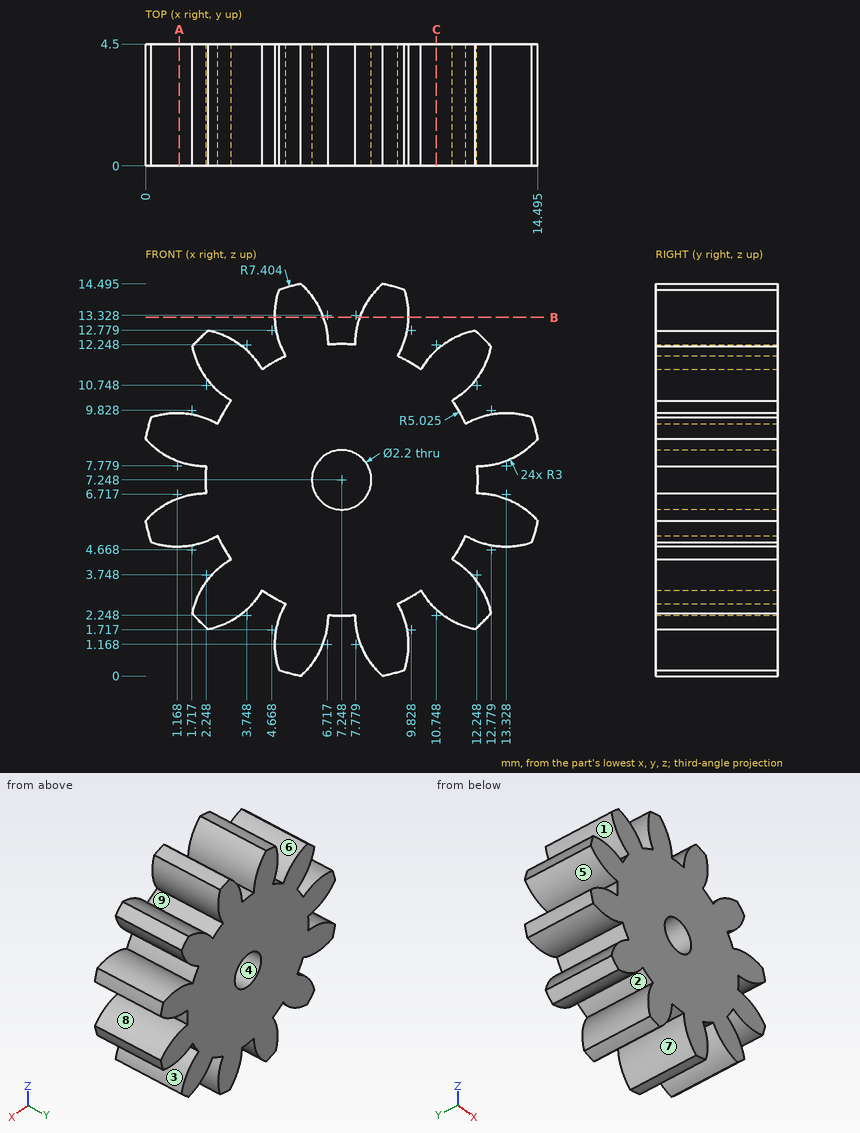
Can you work these out from the drawing? Everything is in mm from the part's minimum corner. A direction names the side the tool comes from. Round coordinates to 2 decimals unless told otherwise and drop trailing zeros. Write each loop counter-clockwise with the first axis right and the second up, starting at its lowest first coordinate (ties: lowest second). Pieces come first, ordered by that corner, then holes. Notation, with made-up numbers: (50, 80.25) - (65, 80.25) arc R13 cw to (65, 88.25) - close; hole circle Ø1 at (10, 51). An arc over 180 degrees is marked (long way). Put each result on its own line as item: value. Start each with the question number.
(1) Thinking about a two-plate mould opening in X: for the marked faces 1, 2, 3 and 4, which applies, released by +X, released by -X, zero draft, split by the parting line, or undercut?
(2) I want a section at A-A, the plane x = 1.25. Please give me the cut outline in (y, z) (1 decimal).
(3) I want a section at C-C, the plane x = 10.75. Please give me the cut outline in (y, z), plus the area to 3 significant figures.
(4) For the marked faces 5, 6, 7, 8 and 9, which set-ups out of +Z, -Z, +X, -X, +Y, -Y let a thin tool reach every point of the face, with its end or its side?
(5) I want a section at B-B, the plane z = 13.25. Please give me the cut outline in (x, y) (1 decimal).
(6) Will this pin go through, and if not, where does the flat tip stop? pin 1 (2 mm diameter, centred on x = 7, y = 3.5, fed in from -Z) (1 decimal).
(7) I need wall thicknesses on probe 1 along Z at (x, y) = (2, 3.8) (1 decimal); probe 2 along X at (y, z) = (2.2, 7.5); probe 3 along Z at (x, y) = (13.25, 1.35) (1 decimal). Which ranges of each line are inside material? Lowest first, please.
Here are the results:
1. face 1: released by -X
1. face 2: undercut
1. face 3: released by +X
1. face 4: undercut
2. outline: (0, 4.8) - (4.5, 4.8) - (4.5, 6.6) - (0, 6.6) - close; (0, 7.9) - (4.5, 7.9) - (4.5, 9.7) - (0, 9.7) - close
3. outline: (0, 2.46) - (4.5, 2.46) - (4.5, 12.04) - (0, 12.04) - close
3. area: 43.1 mm^2
4. face 5: -X, +Y, -Y
4. face 6: +Z, +Y, -Y
4. face 7: -Z, +Y, -Y
4. face 8: +X, +Y, -Y
4. face 9: +Y, -Y
5. outline: (4.8, 0) - (6.6, 0) - (6.6, 4.5) - (4.8, 4.5) - close; (7.9, 0) - (9.7, 0) - (9.7, 4.5) - (7.9, 4.5) - close
6. pin 1: stops at z = 0.3
7. probe 1: z = 2 to 3.1, 4.9 to 6.7, 7.8 to 9.6, 11.4 to 12.5
7. probe 2: x = 2.23 to 6.18, 8.32 to 12.27
7. probe 3: z = 4.8 to 6.6, 7.9 to 9.7
